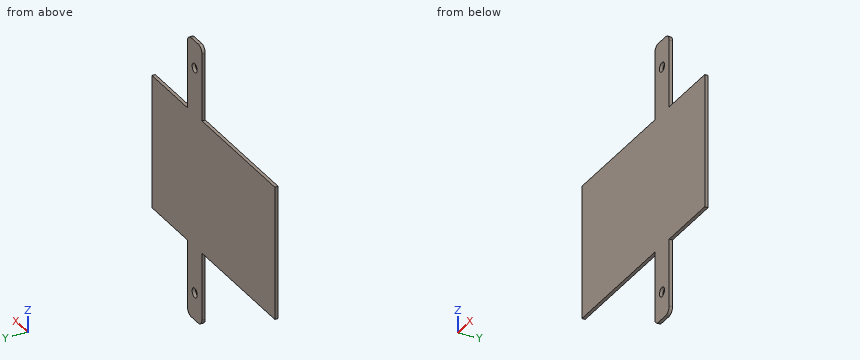
from build123d import *

# Parameters (mm, degrees)
SKETCH1_R           = 7
BOSS_EXTRUDE1_DEPTH = 5


with BuildPart() as part:
    # Sketch1 → Boss-Extrude1 (new body)
    with BuildSketch(Plane(origin=(0, 0, 0), x_dir=(1, 0, 0), z_dir=(0, 1, 0))):
        with BuildLine():
            Line((-449.708642176, 422.631578947), (-351.296475424, 422.631578947))
            Line((-351.296475424, 422.631578947), (-351.296475424, 222.631578947))
            Line((-351.296475424, 222.631578947), (-449.708642176, 222.631578947))
            Line((-449.708642176, 222.631578947), (-449.708642176, 121.631578947))
            ThreePointArc((-449.708642176, 121.631578947), (-452.637574364, 114.560511136), (-459.708642176, 111.631578947))
            Line((-459.708642176, 111.631578947), (-479.708642176, 111.631578947))
            ThreePointArc((-479.708642176, 111.631578947), (-486.779709988, 114.560511136), (-489.708642176, 121.631578947))
            Line((-489.708642176, 121.631578947), (-489.708642176, 222.631578947))
            Line((-489.708642176, 222.631578947), (-691.296475424, 222.631578947))
            Line((-691.296475424, 222.631578947), (-691.296475424, 422.631578947))
            Line((-691.296475424, 422.631578947), (-489.708642176, 422.631578947))
            Line((-489.708642176, 422.631578947), (-489.708642176, 523.631578947))
            ThreePointArc((-489.708642176, 523.631578947), (-486.779709988, 530.702646759), (-479.708642176, 533.631578947))
            Line((-479.708642176, 533.631578947), (-459.708642176, 533.631578947))
            ThreePointArc((-459.708642176, 533.631578947), (-452.637574364, 530.702646759), (-449.708642176, 523.631578947))
            Line((-449.708642176, 523.631578947), (-449.708642176, 422.631578947))
        make_face()
        with Locations((-469.708642176, 492.631578947)):
            Circle(SKETCH1_R, mode=Mode.SUBTRACT)
        with Locations((-469.708642176, 152.631578947)):
            Circle(SKETCH1_R, mode=Mode.SUBTRACT)
    extrude(amount=BOSS_EXTRUDE1_DEPTH)


solid = part.part
Could you check a few things on this model? Use its own coordinates, in mm. Give positions to 0.01 mm unless a question says otherwise; leave off trailing zeros. Order: outer loops, then holes, each group sorted by start corner. A loop starts at its lowest first (then second) coordinate and runs counter-clockwise, first axis right, second up. Notation, with made-up numbers: (66.5, -6) -> (83.5, -6) arc R29 cw to (83.5, 19) -> close; hole circle Ø7 at (-19, -22.5). An arc over 180 degrees is marked (long way). Return JSON: item names as keys, results as strings.
1. Imagine slicing it at A-A on y = 1. List the corners of the cut face in (x, z) for me.
Answer list:
{"outline": "(-691.3, -422.63) -> (-489.71, -422.63) -> (-489.71, -523.63) arc R10 ccw to (-479.71, -533.63) -> (-459.71, -533.63) arc R10 ccw to (-449.71, -523.63) -> (-449.71, -422.63) -> (-351.3, -422.63) -> (-351.3, -222.63) -> (-449.71, -222.63) -> (-449.71, -121.63) arc R10 ccw to (-459.71, -111.63) -> (-479.71, -111.63) arc R10 ccw to (-489.71, -121.63) -> (-489.71, -222.63) -> (-691.3, -222.63) -> close; hole circle Ø14 at (-469.71, -492.63); hole circle Ø14 at (-469.71, -152.63)"}
2. For pin 1 Ø2.5 at (x, y) = (-626.5, 3.5) entering from +Z; pin 2 Ø1 at (x, y) = (-589.5, 4) entering from -Z, each with a flat end and sliding along its axis, tell me the tip position at first contact or that it passes through.
Answer list:
{"pin 1": "stops at z = -222.63", "pin 2": "stops at z = -422.63"}
3. Imagine slicing it at C-C on z = -165. List the corners of the cut face in (x, y) for me, then the cut area to 3 significant figures.
Answer list:
{"outline": "(-489.71, 0) -> (-449.71, 0) -> (-449.71, 5) -> (-489.71, 5) -> close", "area": "200 mm2"}
4. I need wall thicknesses on line 1 (Z direction, x = -415, y = 2.25); line 2 (X direction, y = 4.6, z = -426). Which ranges of each line are inside material? Lowest first, please. Write a range as from..to.
Answer list:
{"line 1": "z = -422.63..-222.63", "line 2": "x = -489.71..-449.71"}
5. Imagine slicing it at B-B on x = -469. List the corners of the cut face in (y, z) for me, then the cut area to 3 significant figures.
Answer list:
{"outline": "(0, -533.63) -> (5, -533.63) -> (5, -499.6) -> (0, -499.6) -> close; (0, -485.67) -> (5, -485.67) -> (5, -159.6) -> (0, -159.6) -> close; (0, -145.67) -> (5, -145.67) -> (5, -111.63) -> (0, -111.63) -> close", "area": "1,970 mm2"}
6. Imagine slicing it at D-D on x = -413.5. List the corners of the cut face in (y, z) for me.
Answer list:
{"outline": "(0, -422.63) -> (5, -422.63) -> (5, -222.63) -> (0, -222.63) -> close"}
